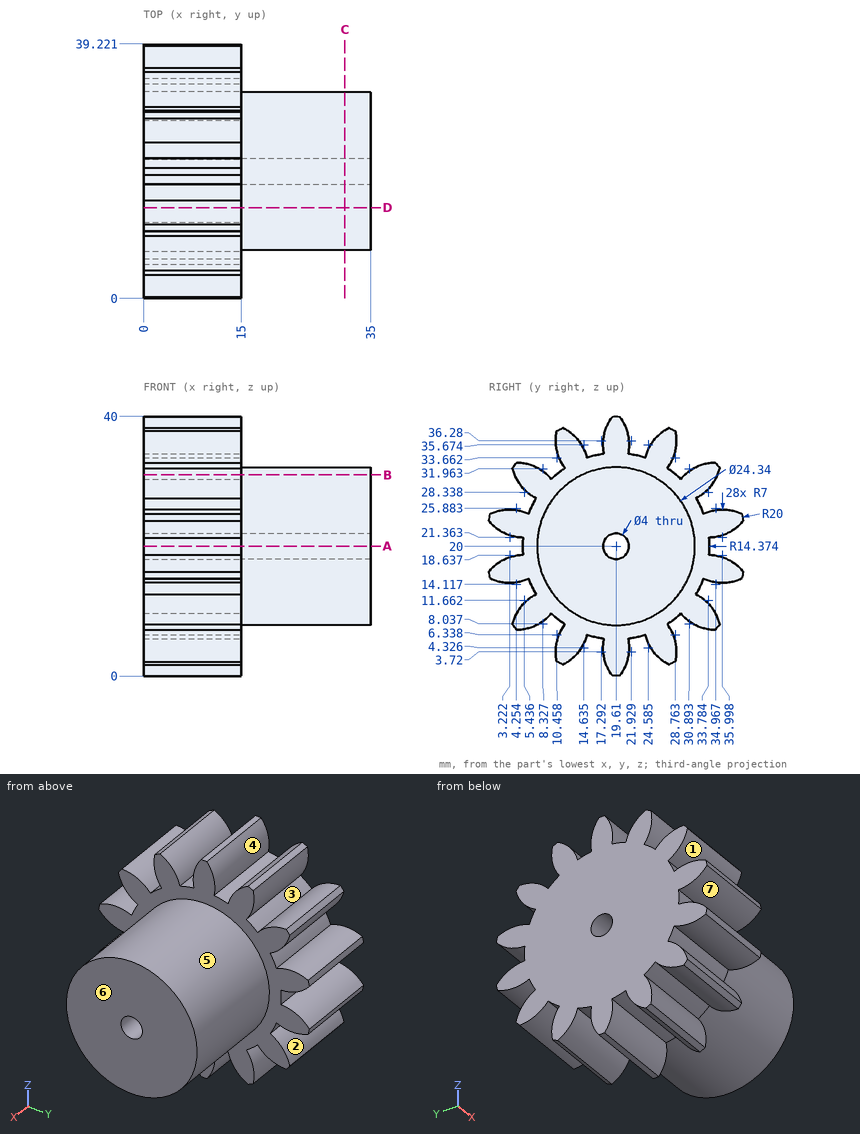
Design review of the part shown in the three views and the two pictorial views. Dimensions are in mm from the part's minimum x, y and z. A direction names the side the tool comes from. Coordinates: 2 decimals unless noted, no trailing zeros. Order: outer loops, then holes, each group sorted by start corner. A loop starts at its lowest first (then second) coordinate and runs counter-clockwise, first axis right, second up.
1) Take a section at C-C, the plane x = 31. Give the boundary of the cut face in (y, z).
2) Take a section at B-B, the plane z = 31. Give the boundary of the cut face in (x, y), and give its area (3 significant figures).
3) Take a section at A-A, the plane z = 20. Give the boundary of the cut face in (x, y) (1 decimal), and give its area (3 significant figures).
4) For the marked faces 1, 2 and 3, list the 3-axis set-ups (+Z, -Z, +X, -X, +Y, -Y) from which the entire face can be reached by the end or side of a thin tool; tool diameter is ignored.
5) Wall thickness on line 1 along Z through (x, y) = (31.5, 19.5); line 2 along Y through (x, z) = (21, 20); line 3 along X through (y, z) = (10, 10.5): over which ranges is each line inside the solid? List them lowest first.
6) Mouldability with a two-part tool opening along Y and no side actions: class the marked faces 4, 5, 6 and 7 as +Y half, -Y half, draft (parallel to the pull), parting line (faces both ways), or undercut.
7) Take a section at D-D, the plane y = 14. Give the boundary of the cut face in (x, z) (1 decimal), and give its area (3 significant figures).
8) Clearance check with flat-ended pins moving along their axes: pin 1 (2 mm diameter, centred on x = 21.5, z = 19.5, fed in from -Y); pin 2 (10 mm diameter, centred on x = 10.5, y = 26.5, fed in from +Z) (1 decimal); pin 3 (1.5 mm diameter, centred on x = 27, z = 23.5, fed in from +Y) (1 decimal). State where each tip first meets the part, or that it passes through.
Returned:
1. outline: circle Ø24.34 at (19.61, 20); hole circle Ø4 at (19.61, 20)
2. outline: (0, 3.98) - (15, 3.98) - (15, 9.03) - (0, 9.03) - close; (0, 10.36) - (15, 10.36) - (15, 14.4) - (35, 14.4) - (35, 24.82) - (15, 24.82) - (15, 28.86) - (0, 28.86) - close; (0, 30.19) - (15, 30.19) - (15, 35.24) - (0, 35.24) - close
2. area: 637 mm2
3. outline: (0, 5.2) - (15, 5.2) - (15, 7.4) - (35, 7.4) - (35, 17.6) - (0, 17.6) - close; (0, 21.6) - (35, 21.6) - (35, 31.8) - (15, 31.8) - (15, 34) - (0, 34) - close
3. area: 778 mm2
4. face 1: +X, -X, -Y
4. face 2: +X, -X, +Y
4. face 3: +X, -X
5. line 1: z = 7.83 to 18, 22 to 32.17
5. line 2: y = 7.44 to 17.61, 21.61 to 31.78
5. line 3: x = 0 to 15
6. face 4: undercut
6. face 5: parting line
6. face 6: draft
6. face 7: -Y half
7. outline: (0, 3.9) - (15, 3.9) - (15, 9.2) - (35, 9.2) - (35, 30.8) - (15, 30.8) - (15, 36.1) - (0, 36.1) - close
7. area: 914 mm2
8. pin 1: stops at y = 7.44
8. pin 2: stops at z = 38.2
8. pin 3: stops at y = 31.5
